Could you check a few things on this model? Use its own coordinates, in mm. A direction names the side the tool comes from. Round coordinates to 2 decimals unless told otherwise and drop trailing zeros. Write each loop counter-clockwise with the first axis right and the second up, starting at its lowest first coordinate (ties: lowest second). Pieces come first, ordered by that corner, then holes. Notation, with made-up numbers: (-12.5, 6.5) -> (16.5, 6.5) arc R10 ccw to (16.5, 18.5) -> close; hole circle Ø2 at (-24.5, 58). An arc over 180 degrees is marked (long way). Return JSON: item names as keys, results as strings.
from build123d import *

# Parameters (mm, degrees)
F0_R     = 7
F1_DEPTH = 5
F2_R     = 1.1
F3_DEPTH = 5.001
F4_R     = 4
F5_DEPTH = 12
F6_SIZE  = 1


with BuildPart() as f1:
    # F0 (on Front) → F1 (new body)
    with BuildSketch(Plane.XZ):
        Circle(F0_R)
    extrude(amount=F1_DEPTH)

    # F2 (on face) → F3 (cut, through all)
    with BuildSketch(Plane.XZ.offset(5)):
        Circle(F2_R)
    extrude(amount=-F3_DEPTH, mode=Mode.SUBTRACT)

    # F4 (on face) → F5 (join)
    with BuildSketch(Plane.XZ.offset(5)):
        Circle(F4_R)
    extrude(amount=F5_DEPTH)

    # F6
    f6_edges = [f1.edges().sort_by_distance(p)[0] for p in [
        (-4, -17, 0),
        (-4, -5, 0),
    ]]
    chamfer(f6_edges, length=F6_SIZE)


solid = f1.part
1) I want a section at B-B, the plane y = -2.75. Please give me the cut outline in (x, z), and give its area (3 significant figures).
Return value:
{"outline": "circle Ø14 at (0, 0); hole circle Ø2.2 at (0, 0)", "area": "150 mm²"}
2) If I drill on probe 1 along Z at (x, y) = (0, -1.8); probe 2 along Y at (x, z) = (4.25, -2.75); probe 3 along X at (y, z) = (-5.75, 0.5), over which ranges is the centre line in solid material (lowest first)? Write a range as [from, to].
Return value:
{"probe 1": "[-7, -1.1], [1.1, 7]", "probe 2": "[-5, 0]", "probe 3": "[-4.22, 4.22]"}
3) I want a section at C-C, the plane z = -5.5. Please give me the cut outline in (x, y), and give its area (3 significant figures).
Return value:
{"outline": "(-4.33, -5) -> (4.33, -5) -> (4.33, 0) -> (-4.33, 0) -> close", "area": "43.3 mm²"}
4) For faces 5 (the face through (1.5, 0, 0.1)), 6 (the face through (-2, -5, 5)), which set-ups out of +Z, -Z, +X, -X, +Y, -Y let a thin tool reach every point of the face, with its end or its side?
Return value:
{"face 5": "+Z, -Z, +X, -X, +Y", "face 6": "-Y"}
5) Will these pins go through, and if not, where does the flat tip stop? pin 1 Ø1.8 at (x, z) = (0, 0.5) entering from +Y; pin 2 Ø6 at (x, y) = (4, -14.5) entering from -Z; pin 3 Ø3 at (x, y) = (1.5, -8) entering from -Z.
Return value:
{"pin 1": "y = 0", "pin 2": "z = -3.87", "pin 3": "z = -4"}
6) I want a section at A-A, the plane x = 0. Please give me the cut outline in (y, z), and give its area (3 significant figures).
Return value:
{"outline": "(-17, -3) -> (-16, -4) -> (-6, -4) -> (-5, -5) -> (-5, -7) -> (0, -7) -> (0, -1.1) -> (-5, -1.1) -> (-5, 1.1) -> (0, 1.1) -> (0, 7) -> (-5, 7) -> (-5, 5) -> (-6, 4) -> (-16, 4) -> (-17, 3) -> close", "area": "155 mm²"}
7) Thinking about a two-plate mould opening in X: for faces 1 (the face through (6.466, -2.465, -2.681)), 2 (the face through (0, -5, 0)), 3 (the face through (1.05, -2.54, 0.33)), 4 (the face through (0, -17, 0)), which applies, pulls with the +X half, pulls with the -X half, needs draft (parallel to the pull), parting line crosses it, or undercut?
Return value:
{"face 1": "parting line crosses it", "face 2": "undercut", "face 3": "undercut", "face 4": "needs draft"}
8) I want a section at D-D, the plane x = -6. Please give me the cut outline in (y, z), and give its area (3 significant figures).
Return value:
{"outline": "(-5, -3.61) -> (0, -3.61) -> (0, 3.61) -> (-5, 3.61) -> close", "area": "36.1 mm²"}
